For this review, take the finished solid that the model builds, in its own axes (mm). Face numbers are marked on the shaded views. A direction names the side the tool comes from. Coordinates: 2 decimals unless noted, no trailing zeros. Write each loop counter-clockwise with the first axis right and the second up, starting at its lowest first coordinate (ties: lowest second). Pieces come first, ordered by that corner, then holes. Notation, with made-up numbers: (-33, -11) -> (25, -11) arc R18 ccw to (25, 20) -> close; hole circle Ø7 at (-8.75, -38.5). An arc over 180 degrees is marked (long way). One line per item, written item: value. Start each with the question number.
1) For probe 1 along X at (y, z) = (-2, 0); probe 2 along X at (y, z) = (-4.5, -14); probe 3 along X at (y, z) = (-2, 7), list the stretches that pass through material, from the lowest coordinate up. Write a range as from..to.
2) Add section B-B (y = -1.5). State the section outline as (x, z) points, and give its area (3 significant figures).
3) Add section A-A (x = 0). State the section outline as (y, z) points, and give its area (3 significant figures).
4) For pin 1 Ø4 at (x, y) = (3.5, 0.5) entering from -Z; pin 2 Ø0.9 at (x, z) = (0.5, -14.5) entering from +Y; pin 3 Ø8 at (y, z) = (-14.5, 15.5) entering from +X; pin 4 Ø12 at (y, z) = (12.5, -13.5) entering from +X, all flat-tipped, find the tip position at first contact; note any pin that passes through.
5) Machinability: for the marked faces 1, 2 and 3, which of the approach directions +Z, -Z, +X, -X, +Y, -Y give a long, thin tool a straight path to every point of the face, cutting with its end or side? Answer none if there is none.
6) Add section D-D (y = 17.5). State the section outline as (x, z) points, and give its area (3 significant figures).
7) Add section C-C (z = 0). State the section outline as (x, y) points, and give its area (3 significant figures).
from build123d import *

# Parameters (mm, degrees)
SKETCH2_R           = 19
BOSS_EXTRUDE2_DEPTH = 35
SKETCH4_R           = 10
BOSS_EXTRUDE3_DEPTH = 5
SKETCH5_R           = 3
BOSS_EXTRUDE4_DEPTH = 16
SKETCH8_W           = 0.5
SKETCH8_H           = 6.116200225
CUT_EXTRUDE2_DEPTH  = 10
SKETCH10_R          = 1.5
CUT_EXTRUDE3_DEPTH  = 7
SKETCH15_R          = 4
BOSS_EXTRUDE5_DEPTH = 22


with BuildPart() as part:
    # Sketch2 → Boss-Extrude2 (new body)
    with BuildSketch(Plane(origin=(0, 0, 0), x_dir=(1, 0, 0), z_dir=(0, 1, 0))):
        with Locations(Location((0, 0, 0), (0, 0, 270))):
            Circle(SKETCH2_R)
    extrude(amount=-BOSS_EXTRUDE2_DEPTH)

    # Sketch4 → Boss-Extrude3 (add)
    with BuildSketch(Plane(origin=(0, 0, 0), x_dir=(1, 0, 0), z_dir=(0, 1, 0))):
        with Locations(Location((0, 0, 0), (0, 0, 270))):
            Circle(SKETCH4_R)
    extrude(amount=BOSS_EXTRUDE3_DEPTH)

    # Sketch5 → Boss-Extrude4 (add)
    with BuildSketch(Plane(origin=(0, 5, 0), x_dir=(1, 0, 0), z_dir=(0, 1, 0))):
        with Locations(Location((0, 0, 0), (0, 0, 270))):
            Circle(SKETCH5_R)
    extrude(amount=BOSS_EXTRUDE4_DEPTH)

    # Sketch8 → Cut-Extrude2 (cut)
    with BuildSketch(Plane(origin=(0, 21, 0), x_dir=(1, 0, 0), z_dir=(0, 1, 0))):
        with Locations((2.75, -0.083275924)):
            Rectangle(SKETCH8_W, SKETCH8_H)
    extrude(amount=-CUT_EXTRUDE2_DEPTH, mode=Mode.SUBTRACT)

    # Sketch10 → Cut-Extrude3 (cut)
    with BuildSketch(Plane(origin=(0, 0, 0), x_dir=(1, 0, 0), z_dir=(0, 1, 0))):
        with Locations(Location((-15, 0, 0), (0, 0, 270))):
            Circle(SKETCH10_R)
        with Locations(Location((0, 14, 0), (0, 0, 270))):
            Circle(SKETCH10_R)
        with Locations(Location((7.5, 12.990381057, 0), (0, 0, 270))):
            Circle(SKETCH10_R)
        with Locations(Location((7.5, -12.990381057, 0), (0, 0, 270))):
            Circle(SKETCH10_R)
        with Locations(Location((12.124355653, -7, 0), (0, 0, 270))):
            Circle(SKETCH10_R)
        with Locations(Location((-12.124355653, -7, 0), (0, 0, 270))):
            Circle(SKETCH10_R)
    extrude(amount=-CUT_EXTRUDE3_DEPTH, mode=Mode.SUBTRACT)

    # Sketch15 → Boss-Extrude5 (add)
    with BuildSketch(Plane.XY):
        with Locations(Location((0, -27, 0), (0, 0, 90))):
            Circle(SKETCH15_R)
    extrude(amount=BOSS_EXTRUDE5_DEPTH)


solid = part.part
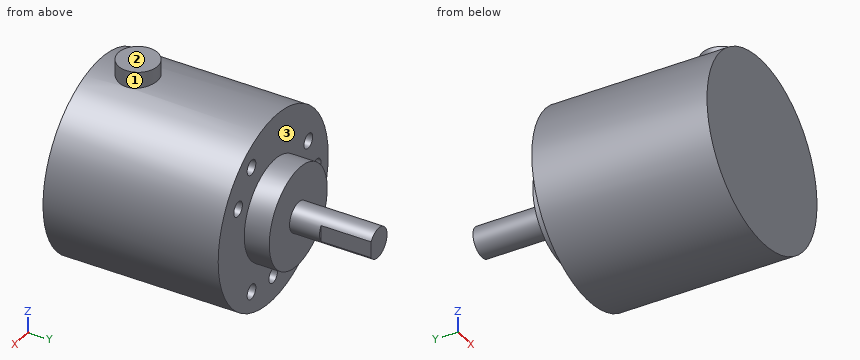
Numbers:
1. probe 1: -19..-16.5, -13.5..19
1. probe 2: -12.85..-1.5, 1.5..6.39, 8.61..12.85
1. probe 3: -17.66..-13.62, -10.62..10.62, 13.62..17.66
2. outline: circle Ø38 at (0, 0); hole circle Ø3 at (-15, 0); hole circle Ø3 at (-12.12, 7); hole circle Ø3 at (0, -14); hole circle Ø3 at (7.5, -12.99); hole circle Ø3 at (7.5, 12.99); hole circle Ø3 at (12.12, 7)
2. area: 1,090 mm²
3. outline: (-35, -19) -> (0, -19) -> (0, -15.5) -> (-7, -15.5) -> (-7, -12.5) -> (0, -12.5) -> (0, -10) -> (5, -10) -> (5, -3) -> (21, -3) -> (21, 3) -> (5, 3) -> (5, 10) -> (0, 10) -> (0, 19) -> (-23, 19) -> (-23, 22) -> (-31, 22) -> (-31, 19) -> (-35, 19) -> close
3. area: 1,530 mm²
4. pin 1: z = -18.94
4. pin 2: y = -7
4. pin 3: x = 15.12
4. pin 4: through
5. face 1: +Z
5. face 2: +Z, +X, -X, +Y, -Y
5. face 3: +Y
6. outline: (2.5, -1.66) -> (2.5, 1.66) arc R3 ccw (long way) to start
6. area: 27.1 mm²
7. outline: (-19, -35) -> (19, -35) -> (19, 0) -> (10, 0) -> (10, 5) -> (3, 5) -> (3, 11) -> (2.5, 11) -> (2.5, 21) -> (-3, 21) -> (-3, 5) -> (-10, 5) -> (-10, 0) -> (-13.5, 0) -> (-13.5, -7) -> (-16.5, -7) -> (-16.5, 0) -> (-19, 0) -> close
7. area: 1,500 mm²
